from build123d import *

# Parameters (mm, degrees)
SKETCH1_R           = 35
SKETCH1_R_2         = 25
BOSS_EXTRUDE1_DEPTH = 90
BOSS_EXTRUDE2_START = -65
SKETCH1_3_R         = 7.5
BOSS_EXTRUDE2_DEPTH = 15
BOSS_EXTRUDE3_START = -15
SKETCH1_4_R         = 15
SKETCH1_4_R_2       = 7.5
BOSS_EXTRUDE3_DEPTH = 15


with BuildPart() as part:
    # Sketch1 → Boss-Extrude1 (new body)
    with BuildSketch(Plane(origin=(0, 0, 0), x_dir=(1, 0, 0), z_dir=(0, 1, 0))):
        with Locations(Location((0, 0, 0), (0, 0, 270))):
            Circle(SKETCH1_R)
        with Locations(Location((0, 0, 0), (0, 0, 270))):
            Circle(SKETCH1_R_2, mode=Mode.SUBTRACT)
    extrude(amount=-BOSS_EXTRUDE1_DEPTH)

    # Sketch1_3 → Boss-Extrude2 (add)
    # profile 1 of 2: a face of its own
    with BuildSketch(Plane(origin=(0, 0, 0), x_dir=(1, 0, 0), z_dir=(0, 1, 0)).offset(BOSS_EXTRUDE2_START)):
        with BuildLine():
            ThreePointArc((8.75, -33.888604279), (-21.433035249, -27.669929526), (-35, 0))
            Line((-35, 0), (-35, -60))
            ThreePointArc((-35, -60), (-5, -90), (25, -60))
            Line((25, -60), (25, -29.692872321))
            Line((25, -29.692872321), (8.75, -33.888604279))
        make_face()
        with Locations(Location((-5, -60, 0), (0, 0, 270))):
            Circle(SKETCH1_3_R, mode=Mode.SUBTRACT)
    # profile 2 of 2: a face of its own
    with BuildSketch(Plane(origin=(0, 0, 0), x_dir=(1, 0, 0), z_dir=(0, 1, 0)).offset(BOSS_EXTRUDE2_START)):
        with BuildLine():
            Line((25, -29.692872321), (25, -24.494897428))
            ThreePointArc((25, -24.494897428), (17.516451042, -30.301385165), (8.75, -33.888604279))
            Line((8.75, -33.888604279), (25, -29.692872321))
        make_face()
    extrude(amount=-BOSS_EXTRUDE2_DEPTH)

    # Sketch1_4 → Boss-Extrude3 (add)
    # profile 1 of 3: a face of its own
    with BuildSketch(Plane(origin=(0, 0, 0), x_dir=(1, 0, 0), z_dir=(0, 1, 0)).offset(BOSS_EXTRUDE3_START)):
        with BuildLine():
            Line((25, -29.692872321), (25, -24.494897428))
            ThreePointArc((25, -24.494897428), (17.516451042, -30.301385165), (8.75, -33.888604279))
            Line((8.75, -33.888604279), (25, -29.692872321))
        make_face()
    # profile 2 of 3: a face of its own
    with BuildSketch(Plane(origin=(0, 0, 0), x_dir=(1, 0, 0), z_dir=(0, 1, 0)).offset(BOSS_EXTRUDE3_START)):
        with BuildLine():
            Line((83.75, 14.523687548), (8.75, 33.888604279))
            ThreePointArc((8.75, 33.888604279), (27.669929526, 21.433035249), (35, 0))
            ThreePointArc((35, 0), (32.403703492, -13.228756555), (25, -24.494897428))
            Line((25, -24.494897428), (25, -29.692872321))
            Line((25, -29.692872321), (83.75, -14.523687548))
            ThreePointArc((83.75, -14.523687548), (65, 0), (83.75, 14.523687548))
        make_face()
    # profile 3 of 3: a face of its own
    with BuildSketch(Plane(origin=(0, 0, 0), x_dir=(1, 0, 0), z_dir=(0, 1, 0)).offset(BOSS_EXTRUDE3_START)):
        with Locations((80, 0)):
            Circle(SKETCH1_4_R)
        with Locations(Location((80, 0, 0), (0, 0, 270))):
            Circle(SKETCH1_4_R_2, mode=Mode.SUBTRACT)
    extrude(amount=-BOSS_EXTRUDE3_DEPTH)


solid = part.part
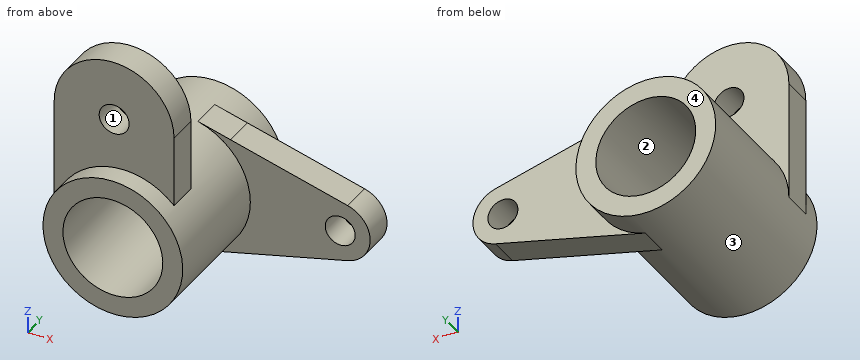
For this review, take the finished solid that the model builds, in its own axes (mm). Face numbers are marked on the shaded views. Round coordinates to 2 decimals unless told otherwise and drop trailing zeros. Order: outer loops, then holes, each group sorted by start corner. A loop starts at its lowest first (then second) coordinate and runs counter-clockwise, first axis right, second up. Notation, with made-up numbers: (-9.75, 8) -> (41.25, 8) arc R10 cw to (41.25, 24) -> close; hole circle Ø7 at (74.5, 62.5). An arc over 180 degrees is marked (long way). Write item = value, one per line. Start each with the question number.
1) Take a section at C-C on x = 16. State the section outline as (y, z) points.
2) Take a section at B-B on x = 0. State the section outline as (y, z) points, plus the area to 3 significant figures.
3) To check wall thickness, follow line 1 (X direction, y = -32, z = 0); line 2 (Y direction, x = 19.5, z = 56); line 3 (Y direction, x = 53, z = -10.5). State the ranges of each line that lie inside material, in increasing order. Write a range as from..to.
4) The part is to be moulded in two halves that separate along Z. For the marked faces 1, 2, 3 and 4, say which applies: +Z half, -Z half, draft (parallel to the pull), parting line (faces both ways), or undercut.
5) Take a section at D-D on z = 70.5. State the section outline as (x, y) points, plus the area to 3 significant figures.
6) Take a section at A-A on y = -67.5. State the section outline as (x, z) points, plus the area to 3 significant figures.
7) Insertion check: pin 1 (10 mm diameter, centred on x = 15.5, y = -9.5, fed in from +Z); pin 2 (12 mm diameter, centred on y = -75, z = 35.5, fed in from +X); pin 3 (18 mm diameter, centred on x = 6.5, z = 38.5, fed in from -Y); pin 4 (6 mm diameter, centred on x = 66.5, y = -18.5, fed in from +Z). Each pin has a flat end and moves straight along its axis. Give the tip position at first contact, or say it passes through.
Verdict:
q1.outline = (-90, -31.13) -> (-30, -31.13) -> (-30, -32.02) -> (-15, -32.02) -> (-15, -31.13) -> (0, -31.13) -> (0, -19.21) -> (-90, -19.21) -> close; (-90, 19.21) -> (0, 19.21) -> (0, 31.13) -> (-15, 31.13) -> (-15, 32.02) -> (-30, 32.02) -> (-30, 31.13) -> (-65, 31.13) -> (-65, 81.42) -> (-80, 81.42) -> (-80, 31.13) -> (-90, 31.13) -> close
q2.outline = (-90, -35) -> (0, -35) -> (0, -25) -> (-90, -25) -> close; (-90, 25) -> (0, 25) -> (0, 35) -> (-65, 35) -> (-65, 54.41) -> (-80, 54.41) -> (-80, 35) -> (-90, 35) -> close; (-80, 65.59) -> (-65, 65.59) -> (-65, 89.58) -> (-80, 89.58) -> close
q2.area = 2,450 mm2
q3.line_1 = -35..-25, 25..35
q3.line_2 = -80..-65
q3.line_3 = -30..-15
q4.face_1 = undercut
q4.face_2 = undercut
q4.face_3 = parting line
q4.face_4 = draft
q5.outline = (-33.1, -80) -> (23.1, -80) -> (23.1, -65) -> (-33.1, -65) -> close
q5.area = 843 mm2
q6.outline = (-35, 0) arc R35 ccw (long way) to (25, 24.49) -> (25, 60) arc R30 ccw to (-35, 60) -> close; hole circle Ø50 at (0, 0); hole circle Ø15 at (-5, 60)
q6.area = 4,970 mm2
q7.pin_1 = 33.39
q7.pin_2 = 25
q7.pin_3 = -90
q7.pin_4 = 19.75
